Could you check a few things on this model? Use its own coordinates, in mm. Face numbers are marked on the shaded views. A direction names the side the tool comes from. Give positions to 0.01 mm unless a question says otherwise; leave off trailing zeros. Order: outer loops, then holes, each group sorted by start corner. A loop starts at its lowest first (then second) coordinate and runs counter-clockwise, first axis right, second up.
(1) Imagine slicing it at A-A, the plane x = 0. Write out the boundary of the cut face in (y, z).
(2) Imagine slicing it at C-C, the plane y = -3.5. State how many separate pieces and enclosed holes the cut face has, then the cut area to 3 significant figures.
(3) If I drill on probe 1 along X at (y, z) = (-2.25, -22); probe 2 along X at (y, z) = (-4.5, 13); probe 3 along X at (y, z) = (-4, 4.5), over which ranges is the centre line in solid material (lowest first)?
(4) On a 3-axis mill with a long thin cutter (end or side, diameter ignored), from which of +Z, -Z, +X, -X, +Y, -Y can I reach the whole of each face in a straight line? I mean the marked faces 1, 2, 3 and 4. Say none if no direction works.
(5) If we mould it in two halves opening along Z, with no side actions, what happens to the marked faces 5, 6 and 7? For each: released by +Z, released by -Z, zero draft, split by the parting line, or undercut.
(6) Will these pins go through, and if not, where does the flat tip stop? pin 1 (2 mm diameter, centred on x = -20, y = -2.5, fed in from +Z); pin 2 (12 mm diameter, centred on x = -7.5, z = -19, fed in from +Y); pin 3 (1.9 mm diameter, centred on y = -1.5, z = -16.5, fed in from -X); pin 4 (1.5 mm diameter, centred on y = -5, z = 14, fed in from -X).
(7) Imagine slicing it at D-D, the plane x = 33.5. Write out the boundary of the cut face in (y, z).
(8) Imagine slicing it at B-B, the plane x = 50.5. Write out the boundary of the cut face in (y, z), then the cut area to 3 significant figures.
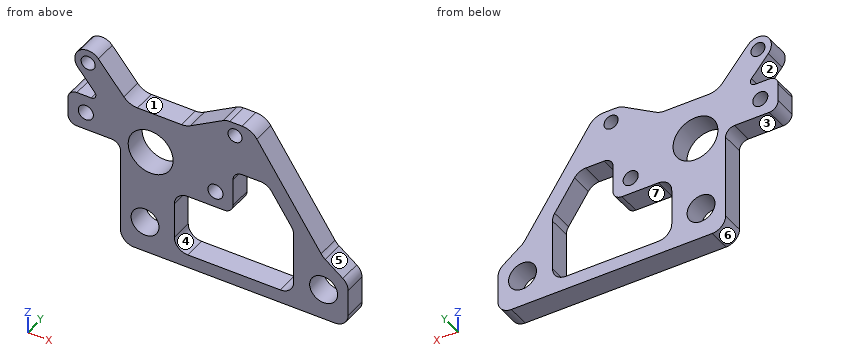
from build123d import *

# Parameters (mm, degrees)
SKETCH4_R           = 6.3881
SKETCH4_R_2         = 3.96875
SKETCH4_R_3         = 2
SKETCH4_R_4         = 2.1463
BOSS_EXTRUDE2_DEPTH = 6.35
FILLET1_R           = 5.08
FILLET7_R           = 3.81
FILLET9_R           = 5.08
FILLET10_R          = 1.27
FILLET11_R          = 3.81
FILLET12_R          = 2.54
FILLET13_R          = 3.81


with BuildPart() as part:
    # Sketch4 → Boss-Extrude2 (new body)
    with BuildSketch(Plane(origin=(0, 0, 0), x_dir=(1, 0, 0), z_dir=(0, 1, 0))):
        with BuildLine():
            Line((28.735494078, -18.4375), (22.483900583, -18.4375))
            ThreePointArc((22.483900583, -18.4375), (21.500464498, -18.308390309), (20.583679925, -17.929811531))
            Line((20.583679925, -17.929811531), (10.16293305, -11.933490986))
            Line((10.16293305, -11.933490986), (-6.103062549, -11.933490986))
            Line((-6.103062549, -11.933490986), (-17.314513469, -25.273959881))
            Line((-17.314513469, -25.273959881), (-23.148009155, -20.371437257))
            Line((-23.148009155, -20.371437257), (-14.139296969, -9.652))
            Line((-14.139296969, -9.652), (-23.52171402, -9.652))
            Line((-23.52171402, -9.652), (-23.52171402, 0.508))
            Line((-23.52171402, 0.508), (-8.5725, 0.508))
            Line((-8.5725, 0.508), (-8.5725, 12.607500122))
            Line((-8.5725, 12.607500122), (-8.5725, 26.9875))
            ThreePointArc((-8.5725, 26.9875), (-7.456576836, 29.681576836), (-4.7625, 30.7975))
            Line((-4.7625, 30.7975), (52.3875, 30.7975))
            ThreePointArc((52.3875, 30.7975), (55.081576836, 29.681576836), (56.1975, 26.9875))
            Line((56.1975, 26.9875), (56.1975, 19.362095927))
            ThreePointArc((56.1975, 19.362095927), (55.797199918, 17.662082259), (54.680415238, 16.319294633))
            Line((54.680415238, 16.319294633), (48.985566477, 12.027918285))
            Line((48.985566477, 12.027918285), (28.735494078, -18.4375))
        make_face()
        with Locations(Location((0, 0, 0), (0, 0, 270))):
            Circle(SKETCH4_R, mode=Mode.SUBTRACT)
        with Locations(Location((-1.5875, 21.9075, 0), (0, 0, 270))):
            Circle(SKETCH4_R_2, mode=Mode.SUBTRACT)
        with Locations(Location((49.2125, 21.9075, 0), (0, 0, 270))):
            Circle(SKETCH4_R_2, mode=Mode.SUBTRACT)
        with Locations(Location((24.012521227, -14.703599027, 0), (0, 0, 270))):
            Circle(SKETCH4_R_3, mode=Mode.SUBTRACT)
        with Locations(Location((-17.78, -19.905950726, 0), (0, 0, 270))):
            Circle(SKETCH4_R_3, mode=Mode.SUBTRACT)
        with Locations(Location((18.44171402, 4.572, 0), (0, 0, 270))):
            Circle(SKETCH4_R_4, mode=Mode.SUBTRACT)
        with Locations(Location((-18.44171402, -4.572, 0), (0, 0, 270))):
            Circle(SKETCH4_R_4, mode=Mode.SUBTRACT)
        Polygon((6.749565973, 26.9875), (40.692955064, 26.9875), (40.692955064, 7.472580753), (33.28904903, -3.666297657), (23.452955064, -3.666297657), (23.452955064, 9.2075), (6.749565973, 9.2075), align=None, mode=Mode.SUBTRACT)
    extrude(amount=-BOSS_EXTRUDE2_DEPTH)

    # Fillet1
    fillet1_edges = [part.edges().sort_by_distance(p)[0] for p in [
        (48.985566477, -3.175, -12.027918285),
        (28.735494078, -3.175, 18.4375),
    ]]
    fillet(fillet1_edges, radius=FILLET1_R)

    # Fillet7
    fillet7_edges = [part.edges().sort_by_distance(p)[0] for p in [
        (40.692955064, -3.175, -7.472580753),
        (40.692955064, -3.175, -26.9875),
        (6.749565973, -3.175, -26.9875),
        (6.749565973, -3.175, -9.2075),
    ]]
    fillet(fillet7_edges, radius=FILLET7_R)

    # Fillet9
    fillet9_edges = [part.edges().sort_by_distance(p)[0] for p in [
        (10.16293305, -3.175, 11.933490986),
        (-6.103062549, -3.175, 11.933490986),
    ]]
    fillet(fillet9_edges, radius=FILLET9_R)

    # Fillet10
    fillet10_edges = [part.edges().sort_by_distance(p)[0] for p in [
        (-14.139296969, -3.175, 9.652),
    ]]
    fillet(fillet10_edges, radius=FILLET10_R)

    # Fillet11
    fillet11_edges = [part.edges().sort_by_distance(p)[0] for p in [
        (-17.314513469, -3.175, 25.273959881),
        (-23.148009155, -3.175, 20.371437257),
    ]]
    fillet(fillet11_edges, radius=FILLET11_R - 0.0001)  # a hair under: the kernel refuses the full size

    # Fillet12
    fillet12_edges = [part.edges().sort_by_distance(p)[0] for p in [
        (23.452955064, -3.175, -9.2075),
        (23.452955064, -3.175, 3.666297657),
        (-23.52171402, -3.175, 9.652),
        (-23.52171402, -3.175, -0.508),
        (-8.5725, -3.175, -0.508),
    ]]
    fillet(fillet12_edges, radius=FILLET12_R)

    # Fillet13
    fillet13_edges = [part.edges().sort_by_distance(p)[0] for p in [
        (33.28904903, -3.175, 3.666297657),
    ]]
    fillet(fillet13_edges, radius=FILLET13_R)


solid = part.part
Answer block:
1. outline: (-6.35, -30.8) - (0, -30.8) - (0, -25.54) - (-6.35, -25.54) - close; (-6.35, -18.27) - (0, -18.27) - (0, -6.39) - (-6.35, -6.39) - close; (-6.35, 6.39) - (0, 6.39) - (0, 11.93) - (-6.35, 11.93) - close
2. separate pieces: 1
2. enclosed holes: 8
2. area: 1,690 mm2
3. probe 1: x = -8.57 to -5.56, 2.38 to 6.75, 40.69 to 45.24, 53.18 to 56.2
3. probe 2: x = -16.95 to -6.85, 12.02 to 22.96, 25.06 to 32.35
3. probe 3: x = -23.52 to -20.59, -16.3 to -4.53, 4.53 to 38
4. face 1: +Z, +Y, -Y
4. face 2: -X, +Y, -Y
4. face 3: -Z, -X, +Y, -Y
4. face 4: +Y, -Y
5. face 5: released by +Z
5. face 6: released by -Z
5. face 7: undercut
6. pin 1: stops at z = 23.52
6. pin 2: stops at y = 0
6. pin 3: stops at x = -8.57
6. pin 4: stops at x = -18.42
7. outline: (-6.35, -30.8) - (0, -30.8) - (0, -26.99) - (-6.35, -26.99) - close; (-6.35, 2.93) - (0, 2.93) - (0, 11.27) - (-6.35, 11.27) - close
8. outline: (-6.35, -30.8) - (0, -30.8) - (0, -25.66) - (-6.35, -25.66) - close; (-6.35, -18.15) - (0, -18.15) - (0, -13.17) - (-6.35, -13.17) - close
8. area: 64.3 mm2
